from build123d import *

# Parameters (mm, degrees)
SKETCH_1_W          = 25
SKETCH_1_H          = 3
EXTRUDE_1_DEPTH     = 3
SKETCH_2_R          = 0.5
CUT_EXTRUDE_1_DEPTH = 4


with BuildPart() as part:
    # 草图1 → 凸台-拉伸1 (new body)
    with BuildSketch(Plane(origin=(0, 0, 0), x_dir=(1, 0, 0), z_dir=(0, 1, 0))):
        Rectangle(SKETCH_1_W, SKETCH_1_H)
    extrude(amount=EXTRUDE_1_DEPTH)

    # 草图2 → 切除-拉伸1 (cut, through all)
    with BuildSketch(Plane(origin=(0, 3, 0), x_dir=(1, 0, 0), z_dir=(0, 1, 0))):
        with Locations((-8, 0)):
            Circle(SKETCH_2_R)
        Circle(SKETCH_2_R)
        with Locations((8, 0)):
            Circle(SKETCH_2_R)
    extrude(amount=-CUT_EXTRUDE_1_DEPTH, mode=Mode.SUBTRACT)


solid = part.part
Verification items for the finished model (mm, model axes). Give positions to 0.01 mm unless a question says otherwise; leave off trailing zeros. Write each loop counter-clockwise with the first axis right and the second up, starting at its lowest first coordinate (ties: lowest second). Pieces come first, ordered by that corner, then holes.
(1) Cross-section at C-C (y = 0.8). Enter the section's corners in (x, z).
(2) Material ranges on line 1 (X direction, y = 2, z = 0); line 2 (Z direction, x = 0, y = 0.65), recorded low to high.
(3) Cross-section at B-B (x = -8). Enter the section's corners in (y, z).
(4) Cross-section at A-A (z = 0). Enter the section's corners in (x, y), plus the area to 3 significant figures.
(5) Mould release check, pull along Z, two halves, no side actions. Record for faces 1 (the face through (-7.523, 1.521, -0.15)), 2 (the face through (12.5, 1, 0)), 3 (the face through (0, 1, 1.5)): +Z half, -Z half, draft (parallel to the pull), parting line (faces both ways), or undercut.
Worked out:
1. outline: (-12.5, -1.5) - (12.5, -1.5) - (12.5, 1.5) - (-12.5, 1.5) - close; hole circle Ø1 at (-8, 0); hole circle Ø1 at (0, 0); hole circle Ø1 at (8, 0)
2. line 1: x = -12.5 to -8.5, -7.5 to -0.5, 0.5 to 7.5, 8.5 to 12.5
2. line 2: z = -1.5 to -0.5, 0.5 to 1.5
3. outline: (0, -1.5) - (3, -1.5) - (3, -0.5) - (0, -0.5) - close; (0, 0.5) - (3, 0.5) - (3, 1.5) - (0, 1.5) - close
4. outline: (-12.5, 0) - (-8.5, 0) - (-8.5, 3) - (-12.5, 3) - close; (-7.5, 0) - (-0.5, 0) - (-0.5, 3) - (-7.5, 3) - close; (0.5, 0) - (7.5, 0) - (7.5, 3) - (0.5, 3) - close; (8.5, 0) - (12.5, 0) - (12.5, 3) - (8.5, 3) - close
4. area: 66.0 mm2
5. face 1: undercut
5. face 2: draft
5. face 3: +Z half
